Geometry check sheet. Reference: the model listing, model coordinates, mm. A direction names the side the tool comes from. Coordinates: 2 decimals unless noted, no trailing zeros. Write each loop counter-clockwise with the first axis right and the second up, starting at its lowest first coordinate (ties: lowest second). Pieces come first, ordered by that corner, then holes. Notation, with made-up numbers: (-21, 61.5) -> (21, 61.5) arc R10 cw to (21, 67.5) -> close; hole circle Ø2 at (-27, -29.75). An arc over 180 degrees is marked (long way). Answer in a Markdown table with one row per item. Add a question column.
Q1. Section check C-C, the plane x = 23.5. Record the boundary of the cut face in (y, z).
Q2. Section check D-D, the plane y = 38.5. Record the boundary of the cut face in (x, z).
Q3. Gauge pin test, flat ends, axial feed: P1, Ø1.6, axis at x = 23, z = 2.5, coming from the +Y side; P2, Ø5, axis at x = 11.5, y = 57, coming from the -Z side; P3, Ø0.9, axis at y = 5, z = 2.5, coming from the -X side; P4, Ø3, axis at y = 21.5, z = 6, coming from the +X side. Record the tip position at first contact, or that the pin passes through.
Q4. Section check A-A, the plane y = 64.16. Record the boundary of the cut face in (x, z) (3 decimals), and give its area (3 significant figures).
Q5. Tool access check on faces 1 (the face through (23, 54.28, 2)), 2 (the face through (22, 4.5, 2)), 3 (the face through (30, 63, 3.5)). Record the directions out of +Z, -Z, +X, -X, +Y, -Y that give a thin tool (end or side, any length) a straight path to the whole face; none if there is none.
Q6. Thickness scan on line 1 (Y direction, x = 35, z = 2.25); line 2 (Y direction, x = 48.92, z = 0.55) (3 decimals); line 3 (X direction, y = 64.16, z = 0.3) (3 decimals). Record the ranges inside material, lowest first.
Q7. Release check for a two-part mould opening along Y. For faces 4 (the face through (34, 9.3, 2)), 5 (the face through (17.8, 46, 2)), 6 (the face through (38.2, 30, 2)) record: pulls with the +Y half, pulls with the -Y half, needs draft (parallel to the pull), parting line crosses it, or undercut.
Q8. Section check B-B, the plane x = 4.42. Record the boundary of the cut face in (y, z) (3 decimals).
```python
from build123d import *

# Parameters (mm, degrees)
SKETCH_1_W      = 53.34
SKETCH_1_H      = 68.58
SKETCH_1_R      = 1.585
EXTRUDE_1_DEPTH = 1.5
SKETCH_2_R      = 3.25
EXTRUDE_2_DEPTH = 8
SKETCH_3_W      = 12
SKETCH_3_H      = 5.3
EXTRUDE_3_DEPTH = 6
SKETCH_4_W      = 2.8
SKETCH_4_H      = 4
EXTRUDE_4_DEPTH = 2
SKETCH_5_W      = 4.8
SKETCH_5_H      = 44
EXTRUDE_5_DEPTH = 4
SKETCH_6_W      = 9
SKETCH_6_H      = 8
EXTRUDE_6_DEPTH = 3
SKETCH_7_W      = 13.1
SKETCH_7_H      = 8.1
SKETCH_7_W_2    = 4.5
SKETCH_7_H_2    = 5.3
SKETCH_7_W_3    = 5.7
SKETCH_7_H_3    = 5.1
SKETCH_7_W_4    = 4.1
SKETCH_7_H_4    = 4.1
SKETCH_7_W_5    = 23
SKETCH_7_H_5    = 23
EXTRUDE_7_DEPTH = 2


with BuildPart() as part:
    # 草图1 → 凸台-拉伸1 (new body)
    with BuildSketch(Plane.XY):
        with Locations((26.67, 34.29)):
            Rectangle(SKETCH_1_W, SKETCH_1_H)
        with Locations((48.92, 64.16)):
            Circle(SKETCH_1_R, mode=Mode.SUBTRACT)
        with Locations((4.42, 64.16)):
            Circle(SKETCH_1_R, mode=Mode.SUBTRACT)
        with Locations((4.42, 4.42)):
            Circle(SKETCH_1_R, mode=Mode.SUBTRACT)
        with Locations((48.92, 4.42)):
            Circle(SKETCH_1_R, mode=Mode.SUBTRACT)
    extrude(amount=EXTRUDE_1_DEPTH)

    # 草图2 → 凸台-拉伸2 (add)
    with BuildSketch(Plane.XY.offset(1.5)):
        with Locations(Location((38.82, 58.16, 0), (0, 0, 180))):
            Circle(SKETCH_2_R)
    extrude(amount=EXTRUDE_2_DEPTH)

    # 草图3 → 凸台-拉伸3 (add)
    with BuildSketch(Plane.XY.offset(1.5)):
        with Locations((32.52, 46.11)):
            Rectangle(SKETCH_3_W, SKETCH_3_H)
    extrude(amount=EXTRUDE_3_DEPTH)

    # 草图4 → 凸台-拉伸4 (add)
    with BuildSketch(Plane.XY.offset(1.5)):
        with Locations((34.44, 11.3)):
            Rectangle(SKETCH_4_W, SKETCH_4_H)
    extrude(amount=EXTRUDE_4_DEPTH)

    # 草图5 → 凸台-拉伸5 (add)
    with BuildSketch(Plane(origin=(0, 0, 0), x_dir=(-1, 0, 0), z_dir=(0, 0, -1))):
        with Locations((-49.04, 34.4)):
            Rectangle(SKETCH_5_W, SKETCH_5_H)
        with Locations((-4.3, 34.4)):
            Rectangle(SKETCH_5_W, SKETCH_5_H)
    extrude(amount=EXTRUDE_5_DEPTH)

    # 草图6 → 凸台-拉伸6 (add)
    with BuildSketch(Plane.XY.offset(1.5)):
        with Locations((40.44, 4)):
            Rectangle(SKETCH_6_W, SKETCH_6_H)
    extrude(amount=EXTRUDE_6_DEPTH)

    # 草图7 → 凸台-拉伸7 (add)
    with BuildSketch(Plane.XY.offset(1.5)):
        with Locations((21.75, 8.55)):
            Rectangle(SKETCH_7_W, SKETCH_7_H)
        with Locations((20.05, 46.03)):
            Rectangle(SKETCH_7_W_2, SKETCH_7_H_2)
        with Locations((23.05, 63.03)):
            Rectangle(SKETCH_7_W_3, SKETCH_7_H_3)
        with Locations((30.45, 63.03)):
            Rectangle(SKETCH_7_W_3, SKETCH_7_H_3)
        with Locations((23.15, 51.73)):
            Rectangle(SKETCH_7_W_3, SKETCH_7_H_3)
        with Locations((30.35, 52.03)):
            Rectangle(SKETCH_7_W_3, SKETCH_7_H_3)
        with Locations((26.85, 57.53)):
            Rectangle(SKETCH_7_W_4, SKETCH_7_H_4)
        with Locations((26.7, 30.6)):
            Rectangle(SKETCH_7_W_5, SKETCH_7_H_5)
    extrude(amount=EXTRUDE_7_DEPTH)


solid = part.part
```
Calculated:
| question | item | result |
|---|---|---|
| 1 | outline | (0, 0) -> (68.58, 0) -> (68.58, 1.5) -> (65.58, 1.5) -> (65.58, 3.5) -> (60.48, 3.5) -> (60.48, 1.5) -> (54.28, 1.5) -> (54.28, 3.5) -> (49.18, 3.5) -> (49.18, 1.5) -> (42.1, 1.5) -> (42.1, 3.5) -> (19.1, 3.5) -> (19.1, 1.5) -> (12.6, 1.5) -> (12.6, 3.5) -> (4.5, 3.5) -> (4.5, 1.5) -> (0, 1.5) -> close |
| 2 | outline | (0, 0) -> (1.9, 0) -> (1.9, -4) -> (6.7, -4) -> (6.7, 0) -> (46.64, 0) -> (46.64, -4) -> (51.44, -4) -> (51.44, 0) -> (53.34, 0) -> (53.34, 1.5) -> (38.2, 1.5) -> (38.2, 3.5) -> (15.2, 3.5) -> (15.2, 1.5) -> (0, 1.5) -> close |
| 3 | P1 | stops at y = 65.58 |
| 3 | P2 | stops at z = 0 |
| 3 | P3 | stops at x = 15.2 |
| 3 | P4 | passes through |
| 4 | outline | (0, 0) -> (2.835, 0) -> (2.835, 1.5) -> (0, 1.5) -> close; (6.005, 0) -> (47.335, 0) -> (47.335, 1.5) -> (33.3, 1.5) -> (33.3, 3.5) -> (27.6, 3.5) -> (27.6, 1.5) -> (25.9, 1.5) -> (25.9, 3.5) -> (20.2, 3.5) -> (20.2, 1.5) -> (6.005, 1.5) -> close; (50.505, 0) -> (53.34, 0) -> (53.34, 1.5) -> (50.505, 1.5) -> close |
| 4 | area | 93.3 mm² |
| 5 | face 1 | +Z, -X |
| 5 | face 2 | +Z, -X, -Y |
| 5 | face 3 | +Z, -X, +Y |
| 6 | line 1 | y = 9.3 to 13.3, 19.1 to 42.1, 43.46 to 48.76 |
| 6 | line 2 | y = 0 to 2.835, 6.005 to 62.575, 65.745 to 68.58 |
| 6 | line 3 | x = 0 to 2.835, 6.005 to 47.335, 50.505 to 53.34 |
| 7 | face 4 | pulls with the -Y half |
| 7 | face 5 | needs draft |
| 7 | face 6 | undercut |
| 8 | outline | (0, 0) -> (2.835, 0) -> (2.835, 1.5) -> (0, 1.5) -> close; (6.005, 0) -> (12.4, 0) -> (12.4, -4) -> (56.4, -4) -> (56.4, 0) -> (62.575, 0) -> (62.575, 1.5) -> (6.005, 1.5) -> close; (65.745, 0) -> (68.58, 0) -> (68.58, 1.5) -> (65.745, 1.5) -> close |
